Read the model definition and answer for the solid it produces. Units are mm, in the model's axes. Give positions to 0.01 mm unless a question says otherwise; leave off trailing zeros. Order: outer loops, then holes, each group sorted by start corner. A loop starts at its lowest first (then second) coordinate and runs counter-clockwise, first axis right, second up. Notation, with made-up numbers: (-28.75, -12.75) - (0.25, -12.75) arc R20 ccw to (0.25, -2.75) - close; hole circle Ø3 at (44.25, 38). An arc over 180 degrees is marked (long way). Return JSON: item names as keys, results as strings.
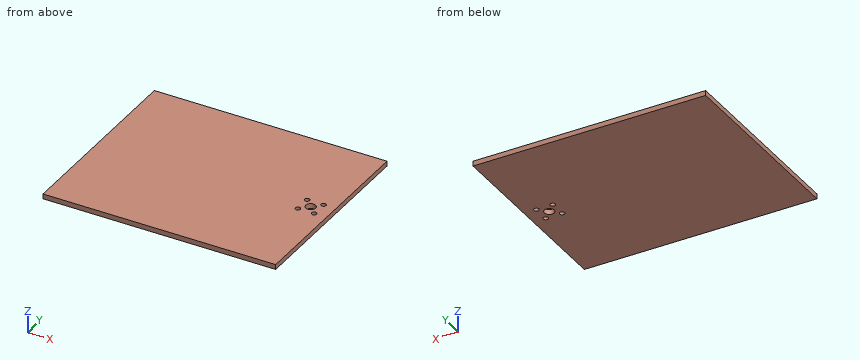
```python
from build123d import *

# Parameters (mm, degrees)
SKETCH_1_W          = 300
SKETCH_1_H          = 118
EXTRUDE_1_DEPTH     = 3
SKETCH_2_R          = 1.5
SKETCH_2_R_2        = 3
CUT_EXTRUDE_1_DEPTH = 3
SKETCH_6_W          = 159
SKETCH_6_H          = 118
CUT_EXTRUDE_2_DEPTH = 10


with BuildPart() as part:
    # 草图1 → 凸台-拉伸1 (new body)
    with BuildSketch(Plane.XY):
        Rectangle(SKETCH_1_W, SKETCH_1_H)
    extrude(amount=EXTRUDE_1_DEPTH)

    # 草图2 → 切除-拉伸1 (cut)
    with BuildSketch(Plane(origin=(0, 0, 0), x_dir=(-1, 0, 0), z_dir=(0, 0, -1))):
        with Locations((-142.449747468, 4.949747468)):
            Circle(SKETCH_2_R)
        with Locations((-132.550252532, 4.949747468)):
            Circle(SKETCH_2_R)
        with Locations((-137.5, 0)):
            Circle(SKETCH_2_R_2)
        with Locations((-142.449747468, -4.949747468)):
            Circle(SKETCH_2_R)
        with Locations((-132.550252532, -4.949747468)):
            Circle(SKETCH_2_R)
    extrude(amount=-CUT_EXTRUDE_1_DEPTH, mode=Mode.SUBTRACT)

    # 草图6 → 切除-拉伸2 (cut)
    with BuildSketch(Plane.XY.offset(3)):
        with Locations((-70.5, 0)):
            Rectangle(SKETCH_6_W, SKETCH_6_H)
    extrude(amount=-CUT_EXTRUDE_2_DEPTH, mode=Mode.SUBTRACT)


solid = part.part
```
Q1. Given pin 1 (1.8 mm diameter, centred on x = 142.45, y = 4.95, fed in from +Z), flat-ended and moving along its own axis, determine where the tip first touches the part or whether it passes through.
Values:
{"pin 1": "passes through"}
Q2. Consider L1, parallel to Y at x = 137.5, z = 2.15; L2, parallel to X at y = -1, z = 1.9. Determine where each line is inside the solid, lowest interval first.
Values:
{"L1": "y = -59 to -3, 3 to 59", "L2": "x = 9 to 134.67, 140.33 to 150"}
Q3. A cutting plane is placed at B-B (y = 0). Write down the section's boundary in (x, z).
Values:
{"outline": "(9, 0) - (134.5, 0) - (134.5, 3) - (9, 3) - close; (140.5, 0) - (150, 0) - (150, 3) - (140.5, 3) - close"}
Q4. A cutting plane is placed at A-A (x = 137.5). Write down the section's boundary in (y, z).
Values:
{"outline": "(-59, 0) - (-3, 0) - (-3, 3) - (-59, 3) - close; (3, 0) - (59, 0) - (59, 3) - (3, 3) - close"}
